Geometry: final body of the model. Coordinates: model frame, mm. A direction names the side the tool comes from. Give positions to 0.01 mm unless a question says otherwise; leave off trailing zeros. Write each loop counter-clockwise with the first axis right and the second up, starting at its lowest first coordinate (ties: lowest second). Pieces come first, ordered by that corner, then holes. Notation, with made-up numbers: (52.25, -19) -> (105.25, -19) arc R22 cw to (105.25, 5) -> close; hole circle Ø4 at (-8.5, 11.5). An arc over 180 degrees is marked (long way). Answer as a JSON object with one key per item and string values.
from build123d import *

# Parameters (mm, degrees)
F0_R      = 3.7211
F1_DEPTH  = 15.24
F3_W      = 11.0588753596
F3_H      = 5.0897249021
F4_DEPTH  = 25.4
F5_R      = 6.35
F5_R_2    = 3.81
F6_DEPTH  = 3.7211
F7_W      = 11.0588753596
F7_H      = 5.0897249021
F8_DEPTH  = 25.4
F9_R      = 6.35
F9_R_2    = 3.81
F10_DEPTH = 3.7211
F11_R     = 3.7211
F12_DEPTH = 1.27


with BuildPart() as f1:
    # F0 (on Top) → F1 (new body)
    with BuildSketch(Plane.XY):
        Circle(F0_R)
    extrude(amount=F1_DEPTH)

    # F3 (on face) → F4 (join)
    with BuildSketch(Plane.XY.offset(15.24)):
        with Locations((5.5294376798, 2.544862451)):
            Rectangle(F3_W, F3_H)
    extrude(amount=F4_DEPTH)

    # F7 (on face) → F8 (cut)
    with BuildSketch(Plane.XY.offset(40.64)):
        with Locations((5.5294376798, 2.544862451)):
            Rectangle(F7_W, F7_H)
    extrude(amount=-F8_DEPTH, mode=Mode.SUBTRACT)



with BuildPart() as f6:
    # F5 (on face) → F6 (new body)
    with BuildSketch(Plane.XZ):
        with Locations((0, 21.59)):
            Circle(F5_R)
        with Locations((0, 21.59)):
            Circle(F5_R_2, mode=Mode.SUBTRACT)
    extrude(amount=F6_DEPTH)


with BuildPart() as f10:
    # F9 (on face) → F10 (new body)
    with BuildSketch(Plane(origin=(0, 0, 0), x_dir=(-1, 0, 0), z_dir=(0, 1, 0))):
        with Locations((0, 21.59)):
            Circle(F9_R)
        with Locations((0, 21.59)):
            Circle(F9_R_2, mode=Mode.SUBTRACT)
    extrude(amount=F10_DEPTH)


with BuildPart() as f1_1:
    add(f1.part)

    add(f6.part)  # F12 merges F6

    add(f10.part)  # F12 merges F10
    # F11 (on face) → F12 (join)
    with BuildSketch(Plane.XY.offset(15.24)):
        Circle(F11_R)
    extrude(amount=F12_DEPTH)


solid = f1_1.part
Q1. Cut plane C-C (y = 2.5). Return the cut outline in (x, z), and give its area (3 significant figures).
Values:
{"outline": "(-2.76, 0) -> (2.76, 0) -> (2.76, 15.87) arc R6.35 ccw (long way) to (-2.76, 15.87) -> close; hole circle Ø7.62 at (0, 21.59)", "area": "166 mm²"}
Q2. Material intervals for L1, parallel to X at y = -1, z = 21.5; L2, parallel to Z at x = 0, y = -2.1; L3, parallel to X at y = 0, z = 12.5, sorted ascending. Write a range as from..to.
Values:
{"L1": "-6.35..-3.81, 3.81..6.35", "L2": "0..17.78, 25.4..27.94", "L3": "-3.72..3.72"}
Q3. Cut plane D-D (z = 2.5). Return the cut outline in (x, y), and give its area (3 significant figures).
Values:
{"outline": "circle Ø7.44 at (0, 0)", "area": "43.5 mm²"}
Q4. First-contact query: P1, Ø3, axis at x = -2.5, y = -1, coming from the +Z side; P2, Ø2, axis at y = -1.5, z = 12, coming from the +X side. Flat tips, straight axial feed; report the tip coordinate or a pass-through.
Values:
{"P1": "z = 27.86", "P2": "x = 3.69"}
Q5. Cut plane B-B (z = 18.25). Return the cut outline in (x, y), and give its area (3 significant figures).
Values:
{"outline": "(-5.4, -3.72) -> (-1.83, -3.72) -> (-1.83, 3.72) -> (-5.4, 3.72) -> close; (1.83, -3.72) -> (5.4, -3.72) -> (5.4, 3.72) -> (1.83, 3.72) -> close", "area": "53.1 mm²"}
Q6. Set-up query: faces 1 (the cylindrical face through (3.437, -1.425, 8.107)), 2 (the flat face through (0, 0, 0)). Return all of +Z, -Z, +X, -X, +Y, -Y with unobstructed straight access to the full face (end or side cutting, diameter ignored); none if empty.
Values:
{"face 1": "-Z", "face 2": "-Z, +X, -X, +Y, -Y"}
Q7. Cut plane A-A (x = -1.25). Return the cut outline in (y, z), and give its area (3 significant figures).
Values:
{"outline": "(-3.72, 15.36) -> (-3.5, 15.36) -> (-3.5, 0) -> (3.5, 0) -> (3.5, 15.36) -> (3.72, 15.36) -> (3.72, 17.99) -> (-3.72, 17.99) -> close; (-3.72, 25.19) -> (3.72, 25.19) -> (3.72, 27.82) -> (-3.72, 27.82) -> close", "area": "147 mm²"}
